from build123d import *

# Parameters (mm, degrees)
F0_W     = 6
F0_H     = 9
F0_R     = 1
F1_DEPTH = 2
F2_W     = 6
F2_H     = 2
F3_DEPTH = 13.5
F4_R     = 1
F5_DEPTH = 25


with BuildPart() as f1:
    # F0 (on Front) → F1 (new body)
    with BuildSketch(Plane.XZ):
        Rectangle(F0_W, F0_H)
        with Locations((0, 1.5)):
            Circle(F0_R, mode=Mode.SUBTRACT)
    extrude(amount=F1_DEPTH)

    # F2 (on face) → F3 (join)
    with BuildSketch(Plane.XZ.offset(2)):
        with Locations((0, -3.5)):
            Rectangle(F2_W, F2_H)
    extrude(amount=F3_DEPTH)

    # F4 (on face) → F5 (cut)
    with BuildSketch(Plane.XY.offset(-2.5)):
        with Locations((0, -12.5)):
            Circle(F4_R)
    extrude(amount=-F5_DEPTH, mode=Mode.SUBTRACT)


solid = f1.part
The model under review builds one solid part; all positions refer to its coordinate system, in mm. A direction names the side the tool comes from. Round coordinates to 2 decimals unless told otherwise and drop trailing zeros. Write each loop counter-clockwise with the first axis right and the second up, starting at its lowest first coordinate (ties: lowest second). Pieces come first, ordered by that corner, then holes. Notation, with made-up numbers: (52, 27) -> (107, 27) arc R15 ccw to (107, 46) -> close; hole circle Ø6 at (27, 15). An arc over 180 degrees is marked (long way). Answer as a JSON object with one key per item and string values.
1. The part is to be moulded in two halves that separate along Y. For faces 3 (the face through (0.46, -13.39, -3.49)), 4 (the face through (0, -15.5, -3)), 5 (the face through (-0.217, -0.986, 0.524)), say which applies: pulls with the +Y half, pulls with the -Y half, needs draft (parallel to the pull), parting line crosses it, or undercut.
Results found:
{"face 3": "undercut", "face 4": "pulls with the -Y half", "face 5": "needs draft"}
2. Machinability: for faces 1 (the face through (0, -2, 0)), 2 (the face through (0, -8, -4.5)), which of the approach directions +Z, -Z, +X, -X, +Y, -Y give a long, thin tool a straight path to every point of the face, cutting with its end or side? Answer none if there is none.
Results found:
{"face 1": "+Z, +X, -X, -Y", "face 2": "-Z, +X, -X, +Y, -Y"}
3. To check wall thickness, follow line 1 along Y through (x, z) = (0, -3.2); line 2 along Z through (x, y) = (0, -1.6); line 3 along Z through (x, y) = (-2.3, -12). State the ranges of each line that lie inside material, in increasing order.
Results found:
{"line 1": "y = -15.5 to -13.5, -11.5 to 0", "line 2": "z = -4.5 to 0.5, 2.5 to 4.5", "line 3": "z = -4.5 to -2.5"}
4. Clearance check with flat-ended pins moving along their axes: pin 1 (2.5 mm diameter, centred on x = 0, z = 1.5, fed in from -Y); pin 2 (1.2 mm diameter, centred on x = 0, y = -12.5, fed in from -Z); pin 3 (1.5 mm diameter, centred on x = -0.5, y = -8, fed in from +Z). State where each tip first meets the part, or that it passes through.
Results found:
{"pin 1": "stops at y = -2", "pin 2": "passes through", "pin 3": "stops at z = -2.5"}
5. We need section A-A on y = -12.5. State the section outline as (x, z) points.
Results found:
{"outline": "(-3, -4.5) -> (-1, -4.5) -> (-1, -2.5) -> (-3, -2.5) -> close; (1, -4.5) -> (3, -4.5) -> (3, -2.5) -> (1, -2.5) -> close"}
6. We need section D-D on y = -1.5. State the section outline as (x, z) points.
Results found:
{"outline": "(-3, -4.5) -> (3, -4.5) -> (3, 4.5) -> (-3, 4.5) -> close; hole circle Ø2 at (0, 1.5)"}
7. We need section C-C on x = 0. State the section outline as (y, z) points.
Results found:
{"outline": "(-15.5, -4.5) -> (-13.5, -4.5) -> (-13.5, -2.5) -> (-15.5, -2.5) -> close; (-11.5, -4.5) -> (0, -4.5) -> (0, 0.5) -> (-2, 0.5) -> (-2, -2.5) -> (-11.5, -2.5) -> close; (-2, 2.5) -> (0, 2.5) -> (0, 4.5) -> (-2, 4.5) -> close"}
8. We need section B-B on z = 1.5. State the section outline as (x, y) points.
Results found:
{"outline": "(-3, -2) -> (-1, -2) -> (-1, 0) -> (-3, 0) -> close; (1, -2) -> (3, -2) -> (3, 0) -> (1, 0) -> close"}
